```python
from build123d import *

# Parameters (mm, degrees)
BOSS_EXTRUDE1_DEPTH = 10
SKETCH2_R           = 3
BOSS_EXTRUDE2_DEPTH = 3


with BuildPart() as part:
    # Sketch1 → Boss-Extrude1 (new body)
    with BuildSketch(Plane(origin=(0, 0, 0), x_dir=(1, 0, 0), z_dir=(0, 1, 0))):
        with BuildLine():
            Line((-24.017268371, 4.839506173), (-15.684746691, 3.160493827))
            ThreePointArc((-15.684746691, 3.160493827), (0, 16), (15.684746691, 3.160493827))
            Line((15.684746691, 3.160493827), (24.017268371, 4.839506173))
            ThreePointArc((24.017268371, 4.839506173), (0, 24.5), (-24.017268371, 4.839506173))
        make_face()
    extrude(amount=BOSS_EXTRUDE1_DEPTH)

    # Sketch2 → Boss-Extrude2 (add)
    with BuildSketch(Plane.XZ):
        with BuildLine():
            Line((37.5, -16), (37.5, 16))
            Line((37.5, 16), (21.748563171, 16))
            ThreePointArc((21.748563171, 16), (12.186057607, 24.093567606), (0, 27))
            ThreePointArc((0, 27), (-27, 0), (0, -27))
            ThreePointArc((0, -27), (12.186057607, -24.093567606), (21.748563171, -16))
            Line((21.748563171, -16), (37.5, -16))
        make_face()
        with Locations(Location((0, 0, 0), (0, 0, 270))):
            Circle(SKETCH2_R, mode=Mode.SUBTRACT)
    extrude(amount=BOSS_EXTRUDE2_DEPTH)


solid = part.part
```
Can you work these out from the model? Positions are in its coordinate system, mm. A direction names the side the tool comes from. Give positions to 0.01 mm unless a question says otherwise; leave off trailing zeros. Order: outer loops, then holes, each group sorted by start corner. A loop starts at its lowest first (then second) coordinate and runs counter-clockwise, first axis right, second up. Notation, with made-up numbers: (83.5, 82) - (127.5, 82) arc R19 cw to (127.5, 89) - close; hole circle Ø7 at (-4.75, 41.5). An arc over 180 degrees is marked (long way). Use a Markdown table: item, result. Add a question column.
Q1. If we mould it in two halves opening along X, with no side actions, what happens to faces 5 (the flat face through (5, -3, 0)), 6 (the flat face through (5, 0, 6)), 7 (the flat face through (-19.91, 4.93, -4.01))? For each: released by +X, released by -X, zero draft, split by the parting line, or undercut.
Q2. On a 3-axis mill with a long thin cutter (end or side, diameter ignored), from which of +Z, -Z, +X, -X, +Y, -Y can I reach the whole of each face in a straight line? I mean faces 1 (the flat face through (30, -1, -16)), 2 (the cylindrical face through (0, 5, -16)), 3 (the flat face through (19.793, 4.93, -3.988)), 4 (the flat face through (30, -1, 16)). Say none if no direction works.
Q3. If we section it at C-C on z = -20: Write out the boundary of the cut face in (x, y).
Q4. If we section it at D-D on y = 2: Write out the boundary of the cut face in (x, z).
Q5. Please list where these lines run through material, in increasing order: line 1 along X through (y, z) = (-1.9, 0); line 2 along X through (y, z) = (6, -11.5); line 3 along Y through (x, z) = (22.5, -10).
Q6. If we section it at A-A on z = 0: Write out the boundary of the cut face in (x, y).
Q7. I'm going to push flat-ended pins straight in: pin 1 (2 mm diameter, centred on x = 13.5, y = 1.5, fed in from -Z); pin 2 (16 mm diameter, centred on x = -7, z = 6, fed in from +Y); pin 3 (2.5 mm diameter, centred on x = 33.5, y = -1.5, fed in from -Z); pin 4 (5 mm diameter, centred on x = 0, z = 0, fed in from -Y). Where does each tip first touch, or does it pass through?
Q8. If we section it at B-B on x = 20.5: Write out the boundary of the cut face in (y, z).
Answers follow:
| question | item | result |
|---|---|---|
| 1 | face 5 | zero draft |
| 1 | face 6 | undercut |
| 1 | face 7 | released by -X |
| 2 | face 1 | -Z, +X, +Y, -Y |
| 2 | face 2 | +Z, +Y |
| 2 | face 3 | +Z, +X, +Y |
| 2 | face 4 | +Z, +X, +Y, -Y |
| 3 | outline | (-18.14, -3) - (18.14, -3) - (18.14, 0) - (14.15, 0) - (14.15, 10) - (-14.15, 10) - (-14.15, 0) - (-18.14, 0) - close |
| 4 | outline | (-24.02, -4.84) arc R24.5 ccw to (24.02, -4.84) - (15.68, -3.16) arc R16 cw to (-15.68, -3.16) - close |
| 5 | line 1 | x = -27 to -3, 3 to 37.5 |
| 5 | line 2 | x = -21.63 to -11.12, 11.12 to 21.63 |
| 5 | line 3 | y = -3 to 0 |
| 6 | outline | (-27, -3) - (-3, -3) - (-3, 0) - (-27, 0) - close; (3, -3) - (37.5, -3) - (37.5, 0) - (3, 0) - close |
| 7 | pin 1 | stops at z = -21.07 |
| 7 | pin 2 | stops at y = 0 |
| 7 | pin 3 | stops at z = -16 |
| 7 | pin 4 | passes through |
| 8 | outline | (-3, -17.57) - (0, -17.57) - (0, -13.42) - (10, -13.42) - (10, -4.13) - (0, -4.13) - (0, 17.57) - (-3, 17.57) - close |
